from build123d import *

# Parameters (mm, degrees)
SKETCH1_W                                         = 279.4
SKETCH1_H                                         = 101.6
SKETCH1_R                                         = 2.15265
SKETCH1_W_2                                       = 6.604
SKETCH1_H_2                                       = 6.35
BOSS_EXTRUDE1_DEPTH                               = 6.604
SKETCH2_R                                         = 2.15265
SKETCH2_W                                         = 6.604
SKETCH2_H                                         = 6.35
CUT_EXTRUDE1_DEPTH                                = 7.604
CSK_FOR_8_FLAT_HEAD_SOCKET_CAP_SCREW1_D           = 4.3053
CSK_FOR_8_FLAT_HEAD_SOCKET_CAP_SCREW1_CSINK_D     = 9.1186
CSK_FOR_8_FLAT_HEAD_SOCKET_CAP_SCREW1_CSINK_ANGLE = 82


with BuildPart() as part:
    # Sketch1 → Boss-Extrude1 (new body)
    with BuildSketch(Plane(origin=(0, 0, 0), x_dir=(0, 0, -1), z_dir=(1, 0, 0))):
        with Locations((0, -50.8)):
            Rectangle(SKETCH1_W, SKETCH1_H)
        with Locations((-133.35, -24.8793)):
            Circle(SKETCH1_R, mode=Mode.SUBTRACT)
        with Locations((-133.35, -76.7207)):
            Circle(SKETCH1_R, mode=Mode.SUBTRACT)
        with Locations((133.35, -24.8793)):
            Circle(SKETCH1_R, mode=Mode.SUBTRACT)
        with Locations((133.35, -76.720700102)):
            Circle(SKETCH1_R, mode=Mode.SUBTRACT)
        with Locations((-133.35, -34.4043)):
            Rectangle(SKETCH1_W_2, SKETCH1_H_2, mode=Mode.SUBTRACT)
        with Locations((-133.35, -15.3543)):
            Rectangle(SKETCH1_W_2, SKETCH1_H_2, mode=Mode.SUBTRACT)
        with Locations((-133.35, -86.2457)):
            Rectangle(SKETCH1_W_2, SKETCH1_H_2, mode=Mode.SUBTRACT)
        with Locations((-133.35, -67.1957)):
            Rectangle(SKETCH1_W_2, SKETCH1_H_2, mode=Mode.SUBTRACT)
        with Locations((133.35, -15.3543)):
            Rectangle(SKETCH1_W_2, SKETCH1_H_2, mode=Mode.SUBTRACT)
        with Locations((133.35, -34.4043)):
            Rectangle(SKETCH1_W_2, SKETCH1_H_2, mode=Mode.SUBTRACT)
        with Locations((133.35, -67.195700102)):
            Rectangle(SKETCH1_W_2, SKETCH1_H_2, mode=Mode.SUBTRACT)
        with Locations((133.35, -86.245700102)):
            Rectangle(SKETCH1_W_2, SKETCH1_H_2, mode=Mode.SUBTRACT)
    extrude(amount=BOSS_EXTRUDE1_DEPTH)

    # Sketch2 → Cut-Extrude1 (cut, through all)
    with BuildSketch(Plane(origin=(6.604, 0, 0), x_dir=(0, 0, -1), z_dir=(1, 0, 0))):
        with Locations((-54.102, -23.622)):
            Circle(SKETCH2_R)
        with Locations((34.798, -55.372)):
            Circle(SKETCH2_R)
        with Locations((-54.102, -55.372)):
            Circle(SKETCH2_R)
        with Locations((34.798, -23.622)):
            Circle(SKETCH2_R)
        with Locations((-54.102, -14.097)):
            Rectangle(SKETCH2_W, SKETCH2_H)
        with Locations((-54.102, -33.147)):
            Rectangle(SKETCH2_W, SKETCH2_H)
        with Locations((34.798, -45.847)):
            Rectangle(SKETCH2_W, SKETCH2_H)
        with Locations((34.798, -64.897)):
            Rectangle(SKETCH2_W, SKETCH2_H)
        with Locations((-54.102, -45.847)):
            Rectangle(SKETCH2_W, SKETCH2_H)
        with Locations((-54.102, -64.897)):
            Rectangle(SKETCH2_W, SKETCH2_H)
        with Locations((34.798, -14.097)):
            Rectangle(SKETCH2_W, SKETCH2_H)
        with Locations((34.798, -33.147)):
            Rectangle(SKETCH2_W, SKETCH2_H)
    extrude(amount=-CUT_EXTRUDE1_DEPTH, mode=Mode.SUBTRACT)

    # CSK for #8 Flat Head Socket Cap Screw1 (through all)
    with Locations(Plane(origin=(6.604, 0, 0), x_dir=(0, 0, -1), z_dir=(1, 0, 0))):
        with Locations((-133.35, -24.8793), (-133.35, -76.7207), (-54.102, -55.372), (-54.102, -23.622), (34.798, -23.622), (34.798, -55.372), (133.35, -76.720700102), (133.35, -24.8793)):
            CounterSinkHole(CSK_FOR_8_FLAT_HEAD_SOCKET_CAP_SCREW1_D / 2, CSK_FOR_8_FLAT_HEAD_SOCKET_CAP_SCREW1_CSINK_D / 2, counter_sink_angle=CSK_FOR_8_FLAT_HEAD_SOCKET_CAP_SCREW1_CSINK_ANGLE)


solid = part.part
Could you check a few things on this model? Use its own coordinates, in mm. A direction names the side the tool comes from. Give positions to 0.01 mm unless a question says otherwise; leave off trailing zeros. One line per question, with ' | ' between items. Start each with the question number.
Item 1: For faces 1 (the conical face through (3.97, -23.345, -135.023)), 2 (the flat face through (3, -83.071, 133)), which set-ups out of +Z, -Z, +X, -X, +Y, -Y let a thin tool reach every point of the face, with its end or its side?
Item 2: I want a section at A-A on x = 1.5. Give the number of separate pieces and of enclosed holes in the cut face, then the cut area to 3 significant figures.
Item 3: Thinking about a two-plate mould opening in Y: for faces 3 (the flat face through (3, 0, 2)), 4 (the flat face through (3, -86, -130.048)), which applies, pulls with the +Y half, pulls with the -Y half, needs draft (parallel to the pull), parting line crosses it, or undercut?
Item 4: I need wall thicknesses on probe 1 along Z at (x, y) = (1.75, -45.5); probe 2 along Z at (x, y) = (3.5, -34); probe 3 along Z at (x, y) = (6.25, -53.5). Which ranges of each line are inside material? Lowest first, please. Write a range as [from, to].
Verdict:
1) face 1: +X | face 2: +X, -X
2) separate pieces: 1 | enclosed holes: 24 | area: 27,600 mm^2
3) face 3: pulls with the +Y half | face 4: undercut
4) probe 1: [-139.7, -38.1], [-31.5, 50.8], [57.4, 139.7] | probe 2: [-139.7, -136.65], [-130.05, -38.1], [-31.5, 50.8], [57.4, 130.05], [136.65, 139.7] | probe 3: [-139.7, -38.62], [-30.98, 50.28], [57.92, 139.7]
